Autodesk Inventor part; units mm, degrees
ref_plane "YZ Plane" through (0, 0, 0) normal (1, 0, 0) x (0, 1, 0)
ref_plane "XZ Plane" through (0, 0, 0) normal (0, 1, 0) x (-1, 0, 0)
ref_plane "XY Plane" through (0, 0, 0) normal (0, 0, 1) x (1, 0, 0)
sketch "_____1" plane through (0, 0, 0) normal (0, 0, 1) x (1, 0, 0)
  line L0 (50, 0) -> (-50, 0)
  line L1 (-4.5, 0) -> (-4.5, 12.55)
  line L2 (-4.5, 12.55) -> (-4.2, 12.55)
  line L3 (-4.2, 12.55) -> (-4.2, 15.95)
  line L4 (-4.2, 15.95) -> (-4.5, 15.95)
  line L5 (-4.5, 15.95) -> (-4.5, 18.2)
  arc A0 (-4.2, 18.5) -> (-4.5, 18.2) centre (-4.2, 18.2) ccw
  line L6 (-4.2, 18.5) -> (2.5, 18.5)
  line L7 (2.5, 18.5) -> (2.5, 20)
  line L8 (2.5, 20) -> (4.5, 20)
  line L9 (4.5, 20) -> (4.5, 15.95)
  line L10 (4.5, 15.95) -> (4.2, 15.95)
  line L11 (4.2, 15.95) -> (4.2, 12.55)
  line L12 (4.2, 12.55) -> (4.5, 12.55)
  line L13 (4.5, 12.55) -> (4.5, 0)
  line L14 (4.5, 0) -> (-4.5, 0)
revolve "Revolution1" add sketch "_____1" angle 360 about axis through (50, 0, 0) along (1, 0, 0)
sketch "_____2" plane through (0, 0, 0) normal (0, 0, 1) x (1, 0, 0)
  line L0 (50, 0) -> (-50, 0)
  line L1 (-4.5, 0) -> (-4.5, 10.3)
  arc A0 (-4.5, 10.3) -> (-4.2, 10) centre (-4.2, 10.3) ccw
  line L2 (-4.2, 10) -> (4.2, 10)
  arc A1 (4.2, 10) -> (4.5, 10.3) centre (4.2, 10.3) ccw
  line L3 (4.5, 10.3) -> (4.5, 0)
  line L4 (4.5, 0) -> (-4.5, 0)
revolve "Revolution2" cut sketch "_____2" angle 360 about axis through (50, 0, 0) along (1, 0, 0)
properties part number "C-FL6904ZZ" material "ステンレス鋼"
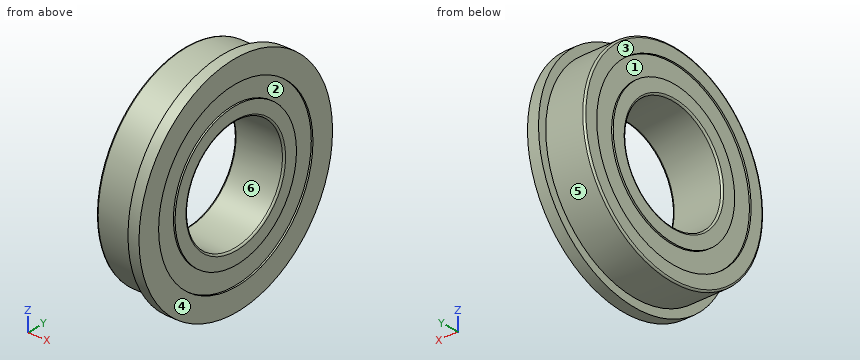
Can you work these out from the model? Positions are in its coordinate system, mm. Face numbers are marked on the shaded views. A direction names the side the tool comes from. Give positions to 0.01 mm unless a question says otherwise; leave off trailing zeros. Write each loop counter-clockwise with the first axis right and the second up, starting at its lowest first coordinate (ties: lowest second). Pieces come first, ordered by that corner, then holes. Notation, with made-up numbers: M -34,-14.5 L 22,-14.5 A25 ccw 22,19.5 Z; hole C 88.5,11 d11. An arc over 180 degrees is marked long. Answer in a Markdown table with one row per item. Add a question column.
Item 1: Please list where these lines run through material, in increasing order: L1, parallel to Z at x = 4.45, y = 0; L2, parallel to X at y = -11, z = -15.5; L3, parallel to X at y = -6.5, z = 13.
Item 2: On a 3-axis mill with a long thin cutter (end or side, diameter ignored), from which of +Z, -Z, +X, -X, +Y, -Y can I reach the whole of each face in a straight line? I mean the marked faces 1, 2 and 3. Say none if no direction works.
Item 3: For pin 1 Ø12 at (y, z) = (1, 1) entering from -X; pin 2 Ø3 at (x, z) = (1.5, 9.5) entering from +Y; pin 3 Ø4 at (x, z) = (-2, -3.5) entering from +Y; pin 4 Ø5 at (x, y) = (-0.5, 12.5) entering from +Z, each with a flat end and sliding along its axis, tell me the tip position at first contact or that it passes through.
Item 4: Imagine slicing it at C-C, the plane x = -0.5. Write out the boundary of the cut face in (y, z).
Item 5: We'd pull the mould along Z, two halves only. Please class the marked faces 4, 5 and 6: released by +Z, released by -Z, zero draft, split by the parting line, or undercut.
Evaluation:
| question | item | result |
|---|---|---|
| 1 | L1 | z = -20 to -15.95, -12.55 to -10.13, 10.13 to 12.55, 15.95 to 20 |
| 1 | L2 | x = 2.5 to 4.5 |
| 1 | L3 | x = -4.2 to 4.2 |
| 2 | face 1 | -X |
| 2 | face 2 | +X |
| 2 | face 3 | +Z, -Z, -X, +Y, -Y |
| 3 | pin 1 | passes through |
| 3 | pin 2 | stops at y = 18.16 |
| 3 | pin 3 | stops at y = 18.44 |
| 3 | pin 4 | stops at z = 15.56 |
| 4 | outline | C 0,0 d37; hole C 0,0 d20 |
| 5 | face 4 | zero draft |
| 5 | face 5 | split by the parting line |
| 5 | face 6 | undercut |
